from build123d import *

# Parameters (mm, degrees)
F1_DEPTH  = 87
F2_R      = 3
F3_R      = 6
F4_R      = 3
F5_R      = 4
F6_W      = 25
F6_H      = 20
F6_R      = 3
F7_DEPTH  = 5
F8_R      = 5
F9_R      = 6
F10_R     = 5.15
F10_R_2   = 6.6
F11_DEPTH = 25
F12_R     = 6.1
F12_R_2   = 3.6
F13_DEPTH = 25
F14_R     = 3
F15_DEPTH = 25


with BuildPart() as f1:
    # F0 (on Front) → F1 (new body)
    with BuildSketch(Plane.XZ):
        Polygon((0, 28), (0, 0), (85, 0), (85, 28), (80, 28), (80, 5), (5, 5), (5, 28), align=None)
    extrude(amount=-F1_DEPTH)

    # F2
    f2_edges = [f1.edges().sort_by_distance(p)[0] for p in [
        (5, 43.5, 5),
    ]]
    fillet(f2_edges, radius=F2_R)

    # F3
    f3_edges = [f1.edges().sort_by_distance(p)[0] for p in [
        (0, 43.5, 0),
        (85, 43.5, 0),
    ]]
    fillet(f3_edges, radius=F3_R)

    # F4
    f4_edges = [f1.edges().sort_by_distance(p)[0] for p in [
        (80, 43.5, 5),
    ]]
    fillet(f4_edges, radius=F4_R)

    # F5
    f5_edges = [f1.edges().sort_by_distance(p)[0] for p in [
        (82.5, 0, 28),
        (2.5, 0, 28),
        (2.5, 87, 28),
        (82.5, 87, 28),
    ]]
    fillet(f5_edges, radius=F5_R)

    # F6 (on face) → F7 (join)
    with BuildSketch(Plane.XY.offset(28)):
        with Locations((72.5, 31)):
            Rectangle(F6_W, F6_H)
        with Locations((67.5, 31)):
            Circle(F6_R, mode=Mode.SUBTRACT)
    extrude(amount=F7_DEPTH)

    # F8
    f8_edges = [f1.edges().sort_by_distance(p)[0] for p in [
        (85, 31, 33),
    ]]
    fillet(f8_edges, radius=F8_R)

    # F9
    f9_edges = [f1.edges().sort_by_distance(p)[0] for p in [
        (60, 21, 30.5),
        (60, 41, 30.5),
    ]]
    fillet(f9_edges, radius=F9_R)

    # F10 (on face) → F11 (cut)
    with BuildSketch(Plane(origin=(0, 0, 0), x_dir=(0, -1, 0), z_dir=(-1, 0, 0))):
        with Locations((-12, 18)):
            Circle(F10_R)
        with Locations((-58, 18)):
            Circle(F10_R_2)
        with Locations((-75, 18)):
            Circle(F10_R)
    extrude(amount=-F11_DEPTH, mode=Mode.SUBTRACT)

    # F12 (on face) → F13 (cut)
    with BuildSketch(Plane.YZ.offset(85)):
        with Locations((75, 18)):
            Circle(F12_R)
        with Locations((58, 18)):
            Circle(F12_R_2)
        with Locations((12, 18)):
            Circle(F12_R)
    extrude(amount=-F13_DEPTH, mode=Mode.SUBTRACT)

    # F14 (on face) → F15 (cut)
    with BuildSketch(Plane(origin=(0, 0, 0), x_dir=(1, 0, 0), z_dir=(0, 0, -1))):
        with Locations((13, -7.5)):
            Circle(F14_R)
        with Locations((13, -25.5)):
            Circle(F14_R)
        with Locations((13, -43.5)):
            Circle(F14_R)
        with Locations((13, -79.5)):
            Circle(F14_R)
        with Locations((13, -61.5)):
            Circle(F14_R)
        with Locations((72, -79.5)):
            Circle(F14_R)
        with Locations((72, -61.5)):
            Circle(F14_R)
        with Locations((72, -43.5)):
            Circle(F14_R)
        with Locations((72, -7.5)):
            Circle(F14_R)
        with Locations((72, -25.5)):
            Circle(F14_R)
    extrude(amount=-F15_DEPTH, mode=Mode.SUBTRACT)


solid = f1.part
Input: part model. Units: mm. Frame: model coordinates. A direction names the side the tool comes from. Give positions to 0.01 mm unless a question says otherwise; leave off trailing zeros. Order: outer loops, then holes, each group sorted by start corner. A loop starts at its lowest first (then second) coordinate and runs counter-clockwise, first axis right, second up. Notation, with made-up numbers: (40.5, 82.5) -> (45.5, 82.5) arc R30 ccw to (45.5, 118.5) -> close; hole circle Ø10 at (84, 22.25). An arc over 180 degrees is marked (long way). Use one line per item in the form item = value.
1) Section B-B, the plane y = 12. Return loops of the section in (x, z), and give its area (3 significant figures).
Response values:
outline = (0, 6) arc R6 ccw to (6, 0) -> (79, 0) arc R6 ccw to (85, 6) -> (85, 11.9) -> (80, 11.9) -> (80, 8) arc R3 cw to (77, 5) -> (8, 5) arc R3 cw to (5, 8) -> (5, 12.85) -> (0, 12.85) -> close; (0, 23.15) -> (5, 23.15) -> (5, 28) -> (0, 28) -> close; (80, 24.1) -> (85, 24.1) -> (85, 28) -> (80, 28) -> close
area = 531 mm^2
2) Section A-A, the plane y = 31. Return loops of the section in (x, z), and give its area (3 significant figures).
Response values:
outline = (0, 6) arc R6 ccw to (6, 0) -> (79, 0) arc R6 ccw to (85, 6) -> (85, 28) arc R5 ccw to (80, 33) -> (70.5, 33) -> (70.5, 28) -> (80, 28) -> (80, 8) arc R3 cw to (77, 5) -> (8, 5) arc R3 cw to (5, 8) -> (5, 28) -> (0, 28) -> close; (60, 28) -> (64.5, 28) -> (64.5, 33) -> (60, 33) -> close
area = 733 mm^2
3) First-contact query: pin 1 Ø4 at (x, y) = (2, 60.5) entering from +Z; pin 2 Ø6 at (x, y) = (54.5, 61.5) entering from +Z; pin 3 Ø9.5 at (x, y) = (13, 25.5) entering from -Z; pin 4 Ø3.5 at (x, y) = (72, 61.5) entering from -Z. Flat tips, straight axial feed; report the tip coordinate or a pass-through.
Response values:
pin_1 = 28
pin_2 = 5
pin_3 = 0
pin_4 = through
4) Section C-C, the plane x = 11.5. Return loops of the section in (y, z), and give its area (3 significant figures).
Response values:
outline = (0, 0) -> (4.9, 0) -> (4.9, 5) -> (0, 5) -> close; (10.1, 0) -> (22.9, 0) -> (22.9, 5) -> (10.1, 5) -> close; (28.1, 0) -> (40.9, 0) -> (40.9, 5) -> (28.1, 5) -> close; (46.1, 0) -> (58.9, 0) -> (58.9, 5) -> (46.1, 5) -> close; (64.1, 0) -> (76.9, 0) -> (76.9, 5) -> (64.1, 5) -> close; (82.1, 0) -> (87, 0) -> (87, 5) -> (82.1, 5) -> close
area = 305 mm^2
5) Reachability of faces 4 (the cylindrical face through (65.1, 29.2, 30.5)), 5 (the cylindrical face through (5.9, 44.11, 5.86)), 6 (the flat face through (83, 62, 28)), 7 (the cylindrical face through (79.14, 44.11, 5.9)) from +Z, -Z, +X, -X, +Y, -Y: full face, straight path, thin tool, end or side. Return the list, or none.
Response values:
face_4 = +Z
face_5 = +Z, +Y, -Y
face_6 = +Z, +X, -X, +Y
face_7 = +Y, -Y
6) Mould query, pull axis X, two halves, no side actions, for faces 1 (the cylindrical face through (83.289, 44.109, 1.804)), 2 (the flat face through (3, 43, 28)), 3 (the flat face through (80, 43, 18)). Classes: pulls with the +X half, pulls with the -X half, needs draft (parallel to the pull), parting line crosses it, or undercut.
Response values:
face_1 = pulls with the +X half
face_2 = needs draft
face_3 = undercut
7) Line query: probe 1 along Y at (x, z) = (72, 2.05); probe 2 along Z at (x, y) = (72, 35); probe 3 along X at (y, z) = (66.5, 24.5). Output: solid intervals per line, ascending.
Response values:
probe_1 = 0 to 4.5, 10.5 to 22.5, 28.5 to 40.5, 46.5 to 58.5, 64.5 to 76.5, 82.5 to 87
probe_2 = 0 to 5, 28 to 33
probe_3 = 0 to 5, 80 to 85
8) Section D-D, the plane y = 53. Return loops of the section in (x, z), and give its area (3 significant figures).
Response values:
outline = (0, 6) arc R6 ccw to (6, 0) -> (79, 0) arc R6 ccw to (85, 6) -> (85, 28) -> (80, 28) -> (80, 8) arc R3 cw to (77, 5) -> (8, 5) arc R3 cw to (5, 8) -> (5, 13.69) -> (0, 13.69) -> close; (0, 22.31) -> (5, 22.31) -> (5, 28) -> (0, 28) -> close
area = 600 mm^2
